For this review, take the finished solid that the model builds, in its own axes (mm). A direction names the side the tool comes from. Coordinates: 2 decimals unless noted, no trailing zeros. Loops run counter-clockwise (first coordinate to the right, second up) from the corner with the lowest first, then second, coordinate; pieces in that order, holes last.
1. To check wall thickness, follow probe 1 along Y at (x, z) = (-21, 41); probe 2 along X at (y, z) = (13.5, -2.5) (3 decimals); probe 3 along X at (y, z) = (0.5, 63.5) (3 decimals). State the ranges of each line that lie inside material, in increasing order.
2. Mouldability with a two-part tool opening along X and no side actions: class faces 6 (the face through (111.12, -0.56, 49.18)), 7 (the face through (56, 0, 42.545)), 8 (the face through (-5, -12.7, 30)) as pulls with the +X half, pulls with the -X half, needs draft (parallel to the pull), parting line crosses it, or undercut.
3. Take a section at A-A, the plane x = 80.5. State the section outline as (y, z) points (3 decimals), then the cut area to 3 significant figures.
4. Machinability: for faces 1 (the face through (41.275, 0, 11)), 2 (the face through (60.325, 0, 37)), 3 (the face through (30.789, 18.961, 52.342)), 4 (the face through (37, -25.4, 21)), 5 (the face through (22.225, -19, 21)), which of the approach directions +Z, -Z, +X, -X, +Y, -Y give a long, thin tool a straight path to every point of the face, cutting with its end or side? Answer none if there is none.
5. Clearance check with flat-ended pins moving along their axes: P1, Ø15.5, axis at x = -10.5, z = 36.5, coming from the +Y side; P2, Ø10, axis at y = -18.5, z = 20, coming from the -X side (3 decimals); P3, Ø6.5, axis at x = -3, y = 20.5, coming from the +Z side (3 decimals). State where each tip first meets the part, or that it passes through.
```python
from build123d import *

# Parameters (mm, degrees)
F1_DEPTH = 25.4
F2_DEPTH = 25.4
F3_DEPTH = 12.7
F0_W     = 25.4
F0_H     = 35.486
F5_R     = 5.08


with BuildPart() as f1:
    # F0 (on Front) → F1 (new body, symmetric)
    with BuildSketch(Plane.XZ):
        Polygon((-41.275, -9.525), (41.275, -9.525), (41.275, 9.525), (22.225, 9.525), (-41.275, 9.525), align=None)
    extrude(amount=F1_DEPTH, both=True)

    # F0 (on Front) → F2 (join, symmetric)
    with BuildSketch(Plane.XZ):
        with BuildLine():
            Line((22.225, 9.525), (41.275, 9.525))
            Line((41.275, 9.525), (41.275, 31.189))
            ThreePointArc((41.275, 31.189), (44.601095, 39.218905), (52.631, 42.545))
            Line((52.631, 42.545), (60.325, 42.545))
            Line((60.325, 42.545), (60.325, 61.595))
            Line((60.325, 61.595), (52.631, 61.595))
            add(Edge.make_bspline(
                [(51.01188, 61.55186), (51.549241, 61.567455), (52.088947, 61.581835), (52.631, 61.595)],
                knots=[106.436193, 106.436193, 106.436193, 106.436193, 107.376077, 107.376077, 107.376077, 107.376077], degree=3))
            ThreePointArc((51.01188, 61.55186), (30.56569, 52.109013), (22.225, 31.189))
            Line((22.225, 31.189), (22.225, 9.525))
        make_face()
        Polygon((60.325, 61.595), (60.325, 42.545), (60.325, 31.189), (85.725, 31.189), (85.725, 66.675), (60.325, 66.675), align=None)
    extrude(amount=F2_DEPTH, both=True)

    # F0 (on Front) → F3 (join, symmetric)
    with BuildSketch(Plane.XZ):
        with BuildLine():
            add(Edge.make_bspline(
                [(-41.275, 9.525), (-40.603282, 42.443589), (-9.840989, 59.785876), (51.01188, 61.55186)],
                knots=[0, 0, 0, 0, 106.436193, 106.436193, 106.436193, 106.436193], degree=3))
            Line((-41.275, 9.525), (22.225, 9.525))
            Line((22.225, 9.525), (22.225, 31.189))
            ThreePointArc((22.225, 31.189), (30.56569, 52.109013), (51.01188, 61.55186))
        make_face()
    extrude(amount=F3_DEPTH, both=True)

    # F0 (on Front) → F4 (revolve)
    with BuildSketch(Plane.XZ):
        with Locations((98.425, 48.932)):
            Rectangle(F0_W, F0_H)
    revolve(axis=Axis((85.725, 0, 48.932), (0, 0, 1)))

    # F5
    f5_edges = [f1.edges().sort_by_distance(p)[0] for p in [
        (-41.275, -25.4, 0),
        (-41.275, 25.4, 0),
    ]]
    fillet(f5_edges, radius=F5_R)


solid = f1.part
```
Results list:
1. probe 1: y = -12.7 to 12.7
1. probe 2: x = -41.275 to 41.275
1. probe 3: x = 60.325 to 111.12
2. face 6: pulls with the +X half
2. face 7: undercut
2. face 8: needs draft
3. outline: (-25.4, 31.189) - (25.4, 31.189) - (25.4, 66.675) - (-25.4, 66.675) - close
3. area: 1,800 mm2
4. face 1: -Z, +X, +Y, -Y
4. face 2: -Z, +Y, -Y
4. face 3: +Z, -X, +Y
4. face 4: +Z, -Z, +X, -X, -Y
4. face 5: +Z, -X, -Y
5. P1: stops at y = 12.7
5. P2: stops at x = 22.225
5. P3: stops at z = 9.525
